```python
from build123d import *

# Parameters (mm, degrees)
F0_R     = 19.05
F1_DEPTH = 3.048
F2_R     = 2.54
F3_R     = 16.678994
F4_DEPTH = 1.651
F5_R     = 7.8105
F6_DEPTH = 4.318
F7_R     = 6.096
F8_DEPTH = 4.191


with BuildPart() as f1:
    # F0 (on Top) → F1 (new body)
    with BuildSketch(Plane.XY):
        Circle(F0_R)
    extrude(amount=F1_DEPTH)

    # F2
    f2_edges = [f1.edges().sort_by_distance(p)[0] for p in [
        (-19.05, 0, 0),
    ]]
    fillet(f2_edges, radius=F2_R)

    # F3 (on face) → F4 (cut)
    with BuildSketch(Plane.XY.offset(3.048)):
        Circle(F3_R)
    extrude(amount=-F4_DEPTH, mode=Mode.SUBTRACT)

    # F5 (on face) → F6 (join)
    with BuildSketch(Plane.XY.offset(1.397)):
        Circle(F5_R)
    extrude(amount=F6_DEPTH)

    # F7 (on face) → F8 (cut)
    with BuildSketch(Plane.XY.offset(5.715)):
        Circle(F7_R)
    extrude(amount=-F8_DEPTH, mode=Mode.SUBTRACT)


solid = f1.part
```
Geometry: final body of the model. Coordinates: model frame, mm. A direction names the side the tool comes from. Give positions to 0.01 mm unless a question says otherwise; leave off trailing zeros. Order: outer loops, then holes, each group sorted by start corner. A loop starts at its lowest first (then second) coordinate and runs counter-clockwise, first axis right, second up. Notation, with made-up numbers: (50.25, 21.25) -> (67.25, 21.25) arc R21 ccw to (67.25, 60.25) -> close; hole circle Ø5 at (21.5, 60). An arc over 180 degrees is marked (long way). Write each question's results on one line, items separated by ' | '. Start each with the question number.
1) Section B-B (z = 4.2). Return loops of the section in (x, y).
2) First-contact query: pin 1 (6 mm diameter, centred on x = -11, y = 1, fed in from -Z); pin 2 (1 mm diameter, centred on y = -0.5, z = 1.5, fed in from +X); pin 3 (3 mm diameter, centred on x = -11, z = 5, fed in from -Y); pin 4 (10 mm diameter, centred on x = 15, y = -13.5, fed in from +Z). Flat tips, straight axial feed; report the tip coordinate or a pass-through.
3) Line query: line 1 (Y direction, x = 0, z = 2.2); line 2 (Y direction, x = 0, z = 1.8); line 3 (X direction, y = -7, z = 2.6). Output: solid intervals per line, ascending. Write a range as from..to.
4) Set-up query: faces 1 (the flat face through (0, 0, 1.524)), 2 (the flat face through (0, 0, 0)). Return all of +Z, -Z, +X, -X, +Y, -Y with unobstructed straight access to the full face (end or side cutting, diameter ignored); none if empty.
5) Draft query along X for faces 3 (the flat face through (5, -4, 5.715)), 4 (the cylindrical face through (-15.12, -11.59, 2.79)), 5 (the cylindrical face through (-0.794, 6.044, 3.649)). Return one class per face: pulls with the +X half, pulls with the -X half, needs draft (parallel to the pull), parting line crosses it, or undercut.
6) Section D-D (z = 0.75). Return loops of the section in (x, y), then the cut area to 3 significant figures.
Calculated:
1) outline: circle Ø15.62 at (0, 0); hole circle Ø12.19 at (0, 0)
2) pin 1: z = 0 | pin 2: x = 18.99 | pin 3: through | pin 4: z = 3.05
3) line 1: -19.03..-16.68, -7.81..-6.1, 6.1..7.81, 16.68..19.03 | line 2: -18.94..-16.68, -7.81..-6.1, 6.1..7.81, 16.68..18.94 | line 3: -17.72..-15.14, -3.46..3.46, 15.14..17.72
4) face 1: +Z | face 2: -Z, +X, -X, +Y, -Y
5) face 3: needs draft | face 4: parting line crosses it | face 5: undercut
6) outline: circle Ø36.62 at (0, 0) | area: 1,050 mm2
